Read the model definition and answer for the solid it produces. Units are mm, in the model's axes. Face numbers are marked on the shaded views. A direction names the side the tool comes from. Give positions to 0.01 mm unless a question says otherwise; leave off trailing zeros. Write each loop counter-clockwise with the first axis right and the second up, starting at its lowest first coordinate (ties: lowest second). Pieces come first, ordered by that corner, then holes. Notation, with made-up numbers: (51.5, 20) -> (84.5, 20) arc R7 ccw to (84.5, 25) -> close; hole circle Ø4 at (85, 21). An arc over 180 degrees is marked (long way). Write item = value, one per line.
from build123d import *

# Parameters (mm, degrees)
BOSS_EXTRUDE1_DEPTH = 88.9
CUT_EXTRUDE1_DEPTH  = 85.09
BOSS_EXTRUDE3_DEPTH = 6.35
SKETCH6_W           = 3.175
SKETCH6_H           = 86.36
CUT_EXTRUDE2_DEPTH  = 3.175
SKETCH7_W           = 86.36
SKETCH7_H           = 76.2
CUT_EXTRUDE3_DEPTH  = 2.54


with BuildPart() as part:
    # Sketch1 → Boss-Extrude1 (new body)
    with BuildSketch(Plane(origin=(0, 0, 0), x_dir=(1, 0, 0), z_dir=(0, 1, 0))):
        with BuildLine():
            Line((0, 0), (0, 88.9))
            Line((0, 88.9), (177.8, 88.9))
            Line((177.8, 88.9), (177.8, 0))
            ThreePointArc((177.8, 0), (88.9, -88.9), (0, 0))
        make_face()
    extrude(amount=BOSS_EXTRUDE1_DEPTH)

    # Sketch2 → Cut-Extrude1 (cut)
    with BuildSketch(Plane(origin=(0, 88.9, 0), x_dir=(1, 0, 0), z_dir=(0, 1, 0))):
        with BuildLine():
            Line((2.54, 88.9), (175.26, 88.9))
            Line((175.26, 88.9), (175.26, 0))
            ThreePointArc((175.26, 0), (90.15621165, -86.692392179), (2.54, -2.54))
            Line((2.54, -2.54), (2.54, 88.9))
        make_face()
    extrude(amount=-CUT_EXTRUDE1_DEPTH, mode=Mode.SUBTRACT)

    # Sketch4 → Boss-Extrude3 (add)
    with BuildSketch(Plane(origin=(177.8, 0, 0), x_dir=(0, 0, -1), z_dir=(1, 0, 0))):
        Polygon((0, 88.9), (88.9, 88.9), (88.9, 0), (0, 0), (0, 6.35), (86.36, 6.35), (86.36, 82.55), (0, 82.55), align=None)
    extrude(amount=BOSS_EXTRUDE3_DEPTH)

    # Sketch6 → Cut-Extrude2 (cut)
    with BuildSketch(Plane(origin=(0, 6.35, 0), x_dir=(1, 0, 0), z_dir=(0, 1, 0))):
        with Locations((180.975, 43.18)):
            Rectangle(SKETCH6_W, SKETCH6_H)
    extrude(amount=-CUT_EXTRUDE2_DEPTH, mode=Mode.SUBTRACT)

    # Sketch7 → Cut-Extrude3 (cut)
    with BuildSketch(Plane(origin=(177.8, 0, 0), x_dir=(0, 0, -1), z_dir=(1, 0, 0))):
        with Locations((43.18, 44.45)):
            Rectangle(SKETCH7_W, SKETCH7_H)
    extrude(amount=-CUT_EXTRUDE3_DEPTH, mode=Mode.SUBTRACT)


solid = part.part
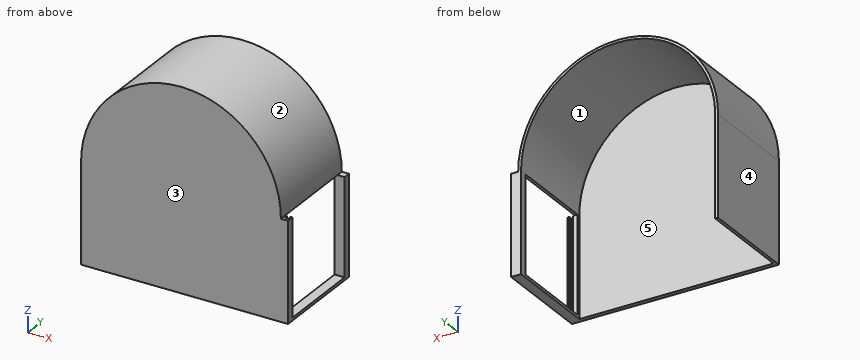
(1) The part is cut by section C-C on x = 88.9. Determine the outline of the cut face in (y, z), plus the area to 3 significant figures.
Checks:
outline = (0, -88.9) -> (3.81, -88.9) -> (3.81, 86.7) -> (88.9, 86.7) -> (88.9, 88.9) -> (0, 88.9) -> close
area = 864 mm²
(2) For a pull along X with two mould halves and no side action, classify the marked faces 1, 2 and 3 as released by +X, released by -X, zero draft, split by the parting line, or undercut.
Checks:
face_1 = undercut
face_2 = split by the parting line
face_3 = zero draft
(3) Consider L1, parallel to Y at x = 168, z = -60; L2, parallel to X at y = 18.5, z = 20; L3, parallel to X at y = 75, z = -50. Determine where each line is inside the solid, lowest interval first.
Checks:
L1 = 0 to 3.81
L2 = 2.28 to 4.78, 172.99 to 175.52
L3 = 0 to 2.54
(4) The part is cut by section D-D on z = 64.5. Determine the outline of the cut face in (x, y), plus the area to 3 significant figures.
Checks:
outline = (27.72, 0) -> (150.08, 0) -> (150.08, 88.9) -> (146.7, 88.9) -> (146.7, 3.81) -> (31.07, 3.81) -> (31.07, 88.9) -> (27.72, 88.9) -> close
area = 1,040 mm²
(5) Given P1, Ø12, axis at x = 158, y = 55, coming from the -Z side; P2, Ø3, axis at x = 123, y = 36, coming from the -Z side; P3, Ø1, axis at y = 55, z = 47.5, coming from the +X side; P4, Ø5, axis at x = 84, z = -23, coming from the -Y side, each flat-ended and moving along its own axis, determine where each tip first touches the part or whether it passes through.
Checks:
P1 = 42.97
P2 = 79.02
P3 = 164.36
P4 = 0
(6) A tool of negligible diameter and unlimited length cuts with its end or side. For the marked faces 4 and 5, from which of +Z, -Z, +X, -X, +Y, -Y can it reach the whole face along a straight path? Write none if from no direction.
Checks:
face_4 = +Z, -Z, -X, +Y, -Y
face_5 = -Z, +Y
